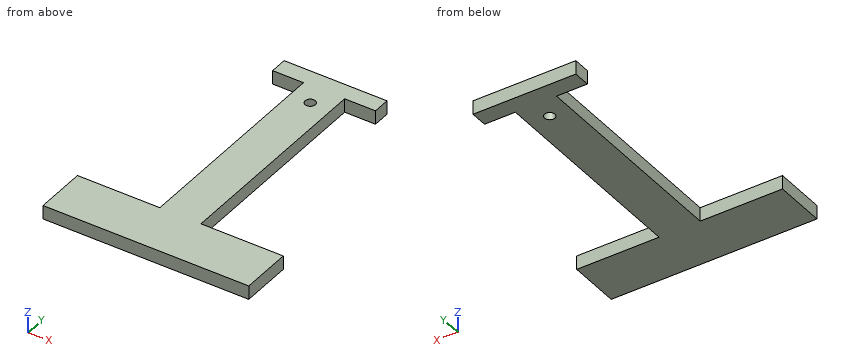
from build123d import *

# Parameters (mm, degrees)
SKETCH_1_R      = 1.5
EXTRUDE_1_DEPTH = 4


with BuildPart() as part:
    # Эскиз1 → Бобышка-Вытянуть1 (new body)
    with BuildSketch(Plane.XY):
        Polygon((5.708165521, 70), (14.708165521, 70), (14.708165521, 75), (-15.291834479, 75), (-15.291834479, 70), (-6.291834479, 70), (-6.291834479, 7.5), (-30.291834479, 7.5), (-30.291834479, -7.5), (29.708165521, -7.5), (29.708165521, 7.5), (5.708165521, 7.5), align=None)
        with Locations((-0.291834479, 64)):
            Circle(SKETCH_1_R, mode=Mode.SUBTRACT)
    extrude(amount=EXTRUDE_1_DEPTH)


solid = part.part
Design review of the part built by this model. Coordinates are the model's own, in mm. Coordinates: 2 decimals unless noted, no trailing zeros. Order: outer loops, then holes, each group sorted by start corner. A loop starts at its lowest first (then second) coordinate and runs counter-clockwise, first axis right, second up. Notation, with made-up numbers: (58, -38.5) -> (108, -38.5) arc R35 ccw to (108, -3.5) -> close; hole circle Ø8 at (-29, 22.5). An arc over 180 degrees is marked (long way). Use one line per item in the form item = value. Start each with the question number.
(1) For probe 1 along X at (y, z) = (64, 1.55); probe 2 along Y at (x, z) = (-11, 2.5); probe 3 along Y at (x, z) = (-27, 2.55), list the stretches that pass through material, from the lowest coordinate up.
(2) Add section C-C on z = 1.4. State the section outline as (x, y) points.
(3) Insertion check: pin 1 (2 mm diameter, centred on x = -20, z = 2.5, fed in from +Y); pin 2 (2.5 mm diameter, centred on x = -0.29, y = 64, fed in from -Z); pin 3 (1.5 mm diameter, centred on y = 19.5, z = 3, fed in from -X); pin 4 (1.2 mm diameter, centred on y = 71.5, z = 1, fed in from +X). Each pin has a flat end and moves straight along its axis. Give the tip position at first contact, or say it passes through.
(4) Add section A-A on y = 64. State the section outline as (x, z) points, plus the area to 3 significant figures.
(5) Add section B-B on x = 11. State the section outline as (y, z) points.
(6) Add section D-D on x = -25.5. State the section outline as (y, z) points.
Answer block:
q1.probe_1 = -6.29 to -1.79, 1.21 to 5.71
q1.probe_2 = -7.5 to 7.5, 70 to 75
q1.probe_3 = -7.5 to 7.5
q2.outline = (-30.29, -7.5) -> (29.71, -7.5) -> (29.71, 7.5) -> (5.71, 7.5) -> (5.71, 70) -> (14.71, 70) -> (14.71, 75) -> (-15.29, 75) -> (-15.29, 70) -> (-6.29, 70) -> (-6.29, 7.5) -> (-30.29, 7.5) -> close; hole circle Ø3 at (-0.29, 64)
q3.pin_1 = 7.5
q3.pin_2 = through
q3.pin_3 = -6.29
q3.pin_4 = 14.71
q4.outline = (-6.29, 0) -> (-1.79, 0) -> (-1.79, 4) -> (-6.29, 4) -> close; (1.21, 0) -> (5.71, 0) -> (5.71, 4) -> (1.21, 4) -> close
q4.area = 36.0 mm²
q5.outline = (-7.5, 0) -> (7.5, 0) -> (7.5, 4) -> (-7.5, 4) -> close; (70, 0) -> (75, 0) -> (75, 4) -> (70, 4) -> close
q6.outline = (-7.5, 0) -> (7.5, 0) -> (7.5, 4) -> (-7.5, 4) -> close
